The model under review builds one solid part; all positions refer to its coordinate system, in mm. Coordinates: 2 decimals unless noted, no trailing zeros. Loops run counter-clockwise (first coordinate to the right, second up) from the corner with the lowest first, then second, coordinate; pieces in that order, holes last. Notation, with made-up numbers: M 24.5,49 L 49.5,49 A24 ccw 49.5,60 Z; hole C 67.25,-7.75 d4. An arc over 180 degrees is marked long. One line per item, written item: value.
```python
from build123d import *

# Parameters (mm, degrees)
SKETCH1_R           = 11.35
SKETCH1_R_2         = 1.65
BOSS_EXTRUDE1_DEPTH = 6.35


with BuildPart() as part:
    # Sketch1 → Boss-Extrude1 (new body)
    with BuildSketch(Plane.XY):
        with BuildLine():
            Line((-31.082201122, 36.863873201), (31.082201122, 36.863873201))
            Line((31.082201122, 36.863873201), (31.082201122, 0.863873201))
            ThreePointArc((31.082201122, 0.863873201), (0, -26.356191916), (-31.082201122, 0.863873201))
            Line((-31.082201122, 0.863873201), (-31.082201122, 36.863873201))
        make_face()
        Circle(SKETCH1_R, mode=Mode.SUBTRACT)
        with Locations((-11.832036089, 7.483510005)):
            Circle(SKETCH1_R_2, mode=Mode.SUBTRACT)
        with Locations((7.483510005, 11.832036089)):
            Circle(SKETCH1_R_2, mode=Mode.SUBTRACT)
        with Locations((11.832036089, -7.483510005)):
            Circle(SKETCH1_R_2, mode=Mode.SUBTRACT)
        with Locations((-7.483510005, -11.832036089)):
            Circle(SKETCH1_R_2, mode=Mode.SUBTRACT)
        with Locations((-25.135580542, 29.363873201)):
            Circle(SKETCH1_R_2, mode=Mode.SUBTRACT)
        with Locations((-17.135580542, 29.363873201)):
            Circle(SKETCH1_R_2, mode=Mode.SUBTRACT)
        with Locations((-9.135580542, 29.363873201)):
            Circle(SKETCH1_R_2, mode=Mode.SUBTRACT)
        with Locations((-1.135580542, 29.363873201)):
            Circle(SKETCH1_R_2, mode=Mode.SUBTRACT)
        with Locations((6.864419458, 29.363873201)):
            Circle(SKETCH1_R_2, mode=Mode.SUBTRACT)
        with Locations((14.864419458, 29.363873201)):
            Circle(SKETCH1_R_2, mode=Mode.SUBTRACT)
        with Locations((22.864419458, 29.363873201)):
            Circle(SKETCH1_R_2, mode=Mode.SUBTRACT)
    extrude(amount=BOSS_EXTRUDE1_DEPTH)


solid = part.part
```
(1) Add section C-C on y = 0. State the section outline as (x, z) points.
Checks:
outline: M -30.95,0 L -11.35,0 L -11.35,6.35 L -30.95,6.35 Z; M 11.35,0 L 30.95,0 L 30.95,6.35 L 11.35,6.35 Z
(2) Draft analysis for pull direction Y (two halves, no side actions). For faces 1 (the face through (22.507, 27.753, 3.131)), 2 (the face through (0, 13, 6.35)), 3 (the face through (0.63, -26.35, 3.13)), state which applies: pulls with the +Y half, pulls with the -Y half, needs draft (parallel to the pull), parting line crosses it, or undercut.
Checks:
face 1: undercut
face 2: needs draft
face 3: pulls with the -Y half
(3) To check wall thickness, follow L1, parallel to X at y = 10.5, z = 2.5; L2, parallel to X at y = -8, z = 2; L3, parallel to X at y = -10, z = 0.5. State the ranges of each line that lie inside material, in increasing order. Write a range as [from, to].
Checks:
L1: [-31.08, -4.31], [4.31, 6.51], [8.46, 31.08]
L2: [-28.53, -8.05], [8.05, 10.26], [13.4, 28.53]
L3: [-27.54, -5.37], [5.37, 27.54]
(4) Add section A-A on x = 12.5. State the section outline as (y, z) points, then the cut area to 3 significant figures.
Checks:
outline: M -23.76,0 L -8.99,0 L -8.99,6.35 L -23.76,6.35 Z; M -5.97,0 L 36.86,0 L 36.86,6.35 L -5.97,6.35 Z
area: 366 mm^2
(5) Add section D-D on y = -15.5. State the section outline as (x, z) points, then the cut area to 3 significant figures.
Checks:
outline: M -23.73,0 L 23.73,0 L 23.73,6.35 L -23.73,6.35 Z
area: 301 mm^2
(6) Add section B-B on z = 2. State how many separate pieces and enclosed holes the cut face has, then the cut area to 3 significant figures.
Checks:
separate pieces: 1
enclosed holes: 12
area: 3,020 mm^2
